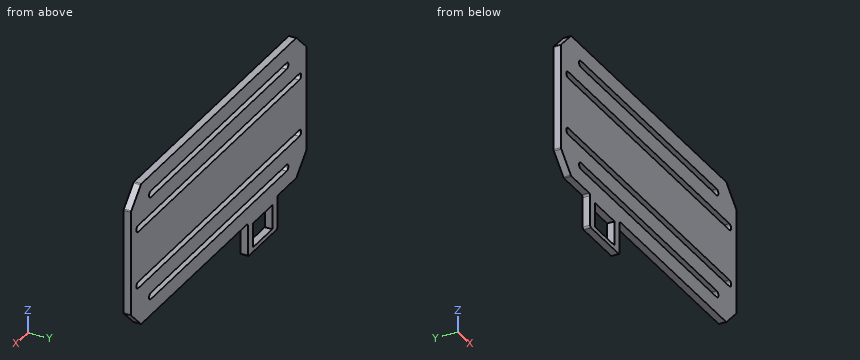
```python
from build123d import *

# Parameters (mm, degrees)
SKETCH2_W           = 174.37
SKETCH2_H           = 77
BOSS_EXTRUDE1_DEPTH = 4
CUT_EXTRUDE1_DEPTH  = 4
SKETCH4_W           = 29.3
SKETCH4_H           = 18.2
SKETCH4_W_2         = 19.3
SKETCH4_H_2         = 13.2
BOSS_EXTRUDE2_DEPTH = 4
CHAMFER1_SIZE       = 10
FILLET1_R           = 1
CUT_EXTRUDE2_DEPTH  = 10


with BuildPart() as part:
    # Sketch2 → Boss-Extrude1 (new body)
    with BuildSketch(Plane(origin=(0, 0, 0), x_dir=(1, 0, 0), z_dir=(0, 1, 0))):
        Rectangle(SKETCH2_W, SKETCH2_H)
    extrude(amount=BOSS_EXTRUDE1_DEPTH)

    # Sketch3 → Cut-Extrude1 (cut)
    with BuildSketch(Plane(origin=(0, 4, 0), x_dir=(1, 0, 0), z_dir=(0, 1, 0))):
        with BuildLine():
            Line((-67.5, 29.75), (67.5, 29.75))
            ThreePointArc((67.5, 29.75), (69.25, 28), (67.5, 26.25))
            Line((67.5, 26.25), (-67.5, 26.25))
            ThreePointArc((-67.5, 26.25), (-69.25, 28), (-67.5, 29.75))
        make_face()
        with BuildLine():
            Line((-67.5, -29.75), (67.5, -29.75))
            ThreePointArc((67.5, -29.75), (69.25, -28), (67.5, -26.25))
            Line((67.5, -26.25), (-67.5, -26.25))
            ThreePointArc((-67.5, -26.25), (-69.25, -28), (-67.5, -29.75))
        make_face()
    extrude(amount=-CUT_EXTRUDE1_DEPTH, mode=Mode.SUBTRACT)

    # Sketch4 → Boss-Extrude2 (add)
    with BuildSketch(Plane.XZ):
        with Locations((-43.5925, -47.6)):
            Rectangle(SKETCH4_W, SKETCH4_H)
        with Locations((-43.5925, -47.6)):
            Rectangle(SKETCH4_W_2, SKETCH4_H_2, mode=Mode.SUBTRACT)
    extrude(amount=-BOSS_EXTRUDE2_DEPTH)

    # Chamfer1
    chamfer1_edges = [part.edges().sort_by_distance(p)[0] for p in [
        (-87.185, 2, -38.5),
        (87.185, 2, -38.5),
        (87.185, 2, 38.5),
        (-87.185, 2, 38.5),
    ]]
    chamfer(chamfer1_edges, length=CHAMFER1_SIZE)

    # Fillet1
    fillet1_edges = [part.edges().sort_by_distance(p)[0] for p in [
        (-58.2425, 2, -56.7),
        (-58.2425, 2, -38.5),
        (-28.9425, 2, -38.5),
        (-28.9425, 2, -56.7),
        (-87.185, 2, 28.5),
        (-87.185, 2, -28.5),
        (-77.185, 2, -38.5),
        (77.185, 2, -38.5),
        (87.185, 2, 28.5),
        (87.185, 2, -28.5),
        (-77.185, 2, 38.5),
        (77.185, 2, 38.5),
    ]]
    fillet(fillet1_edges, radius=FILLET1_R)

    # Sketch5 → Cut-Extrude2 (cut)
    with BuildSketch(Plane(origin=(0, 4, 0), x_dir=(1, 0, 0), z_dir=(0, 1, 0))):
        with BuildLine():
            Line((-80.185, 13.75), (80.185, 13.75))
            ThreePointArc((80.185, 13.75), (81.935, 15.5), (80.185, 17.25))
            Line((80.185, 17.25), (-80.185, 17.25))
            ThreePointArc((-80.185, 17.25), (-81.935, 15.5), (-80.185, 13.75))
        make_face()
        with BuildLine():
            Line((80.185, -17.25), (-80.185, -17.25))
            ThreePointArc((-80.185, -17.25), (-81.935, -15.5), (-80.185, -13.75))
            Line((-80.185, -13.75), (80.185, -13.75))
            ThreePointArc((80.185, -13.75), (81.935, -15.5), (80.185, -17.25))
        make_face()
    extrude(amount=-CUT_EXTRUDE2_DEPTH, mode=Mode.SUBTRACT)


solid = part.part
```
Can you work these out from the model? Positions are in its coordinate system, mm. Coordinates: 2 decimals unless noted, no trailing zeros. Loops run counter-clockwise (first coordinate to the right, second up) from the corner with the lowest first, then second, coordinate; pieces in that order, holes last. Notation, with made-up numbers: M -39.75,17.25 L -23.75,17.25 A25 cw -23.75,45.25 Z; hole C 32.5,11.5 d11. An arc over 180 degrees is marked long. Put each result on its own line as item: value. Start each with the question number.
(1) Imagine slicing it at A-A on x = 8. List the corners of the cut face in (y, z) for me.
(2) Imagine slicing it at B-B on z = -49. List the corners of the cut face in (x, y) for me, and give its area (3 significant figures).
(3) Imagine slicing it at C-C on x = -72. List the corners of the cut face in (y, z) for me, and give its area (3 significant figures).
(4) Will these pins go through, and if not, where does the flat tip stop? pin 1 Ø2 at (x, y) = (23.5, 1.5) entering from -Z; pin 2 Ø2 at (y, z) = (3, -48) entering from +X; pin 3 Ø1.2 at (y, z) = (2.5, -45.5) entering from -X.
(5) I need wall thicknesses on probe 1 along Z at (x, y) = (-72, 3.7); probe 2 along Z at (x, y) = (-27.5, 0.7); probe 3 along Z at (x, y) = (-53, 3.5). Which ranges of each line are inside material? Lowest first, please.
(6) Imagine slicing it at D-D on z = 15.5. List the corners of the cut face in (x, y) for me (3 decimals), and give its area (3 significant figures).
Worked answers:
1. outline: M 0,-38.5 L 4,-38.5 L 4,-29.75 L 0,-29.75 Z; M 0,-26.25 L 4,-26.25 L 4,-17.25 L 0,-17.25 Z; M 0,-13.75 L 4,-13.75 L 4,13.75 L 0,13.75 Z; M 0,17.25 L 4,17.25 L 4,26.25 L 0,26.25 Z; M 0,29.75 L 4,29.75 L 4,38.5 L 0,38.5 Z
2. outline: M -58.24,0 L -53.24,0 L -53.24,4 L -58.24,4 Z; M -33.94,0 L -28.94,0 L -28.94,4 L -33.94,4 Z
2. area: 40.0 mm2
3. outline: M 0,-38.5 L 4,-38.5 L 4,-17.25 L 0,-17.25 Z; M 0,-13.75 L 4,-13.75 L 4,13.75 L 0,13.75 Z; M 0,17.25 L 4,17.25 L 4,38.5 L 0,38.5 Z
3. area: 280 mm2
4. pin 1: stops at z = -38.5
4. pin 2: stops at x = -28.94
4. pin 3: stops at x = -58.24
5. probe 1: z = -38.5 to -17.25, -13.75 to 13.75, 17.25 to 38.5
5. probe 2: z = -38.5 to -29.75, -26.25 to -17.25, -13.75 to 13.75, 17.25 to 26.25, 29.75 to 38.5
5. probe 3: z = -56.7 to -54.2, -41 to -29.75, -26.25 to -17.25, -13.75 to 13.75, 17.25 to 26.25, 29.75 to 38.5
6. outline: M -87.185,0 L -81.935,0 L -81.935,4 L -87.185,4 Z; M 81.935,0 L 87.185,0 L 87.185,4 L 81.935,4 Z
6. area: 42.0 mm2
